Could you check a few things on this model? Use its own coordinates, in mm. A direction names the side the tool comes from. Give positions to 0.01 mm unless a question says otherwise; leave off trailing zeros. Loops run counter-clockwise (first coordinate to the right, second up) from the corner with the lowest first, then second, coordinate; pieces in that order, holes last. Notation, with made-up numbers: (84, 15) -> (96, 15) arc R5 ccw to (96, 21) -> close; hole circle Ø5 at (9.25, 14). An arc over 180 degrees is marked (long way). Write item = value, one per line. Start each with the question number.
1) I want a section at B-B (z = 0.5). List the corners of the cut face in (x, y) for me, and give its area (3 significant figures).
2) I want a section at A-A (y = 0). List the corners of the cut face in (x, z) for me.
3) I need wall thicknesses on probe 1 along Z at (x, y) = (6.5, 11); probe 2 along X at (y, z) = (-8.5, -0.7); probe 3 along X at (y, z) = (3, -1.5). Which ranges of each line are inside material? Lowest first, please. Write a range as from..to.
4) I'm going to push flat-ended pins straight in: pin 1 Ø1 at (x, z) = (1.5, -1) entering from +Y; pin 2 Ø0.6 at (x, z) = (-1, 1.5) entering from +Y. Where does each tip first touch, or does it pass through?
5) I want a section at C-C (x = -8). List the corners of the cut face in (y, z) for me, and give its area (3 significant figures).
6) On a 3-axis mill with a long thin cutter (end or side, diameter ignored), from which of +Z, -Z, +X, -X, +Y, -Y can I reach the whole of each face in a straight line? I mean faces 1 (the face through (3.09, 4.75, -0.94)), 2 (the face through (-11.811, -2.346, -0.937)), 3 (the face through (-5.88, 10.51, -0.94)), 4 (the face through (12.35, 0.37, -0.94)). Say none if no direction works.
7) I want a section at D-D (y = 8.5). List the corners of the cut face in (x, z) for me.
8) If we mould it in two halves opening along X, with no side actions, what happens to faces 5 (the face through (-4.518, 3.136, -0.937)), 6 (the face through (-9.774, -7.56, -0.937)), 7 (the face through (-7, 6, -1.9))? For each: +X half, -X half, draft (parallel to the pull), parting line (faces both ways), or undercut.
from build123d import *

# Parameters (mm, degrees)
SKETCH1_R           = 15.5
BOSS_EXTRUDE1_DEPTH = 2
BOSS_EXTRUDE2_DEPTH = 1.9
CIRPATTERN1_COUNT   = 5
CUT_EXTRUDE2_DEPTH  = 4.9


with BuildPart() as part:
    # Sketch1 → Boss-Extrude1 (new body)
    with BuildSketch(Plane.XY):
        Circle(SKETCH1_R)
    extrude(amount=BOSS_EXTRUDE1_DEPTH)

    # Sketch2 → Boss-Extrude2 (add)
    with BuildSketch(Plane(origin=(0, 0, 0), x_dir=(-1, 0, 0), z_dir=(0, 0, -1))):
        with BuildLine():
            Line((-7.817353518, 8.129035943), (-3.552701535, 4.927044661))
            ThreePointArc((-3.552701535, 4.927044661), (-3.081541521, 4.749426556), (-2.588715364, 4.852685109))
            ThreePointArc((-2.588715364, 4.852685109), (-1.571286021, 5.27077416), (-0.491007267, 5.478039053))
            ThreePointArc((-0.491007267, 5.478039053), (-0.022087339, 5.66148946), (0.274905404, 6.068103848))
            Line((0.274905404, 6.068103848), (2.090121325, 11.082582471))
            ThreePointArc((2.090121325, 11.082582471), (2.007658151, 11.864965509), (1.341576089, 12.283603874))
            ThreePointArc((1.341576089, 12.283603874), (-3.530150602, 11.841654752), (-7.848632729, 9.543883635))
            ThreePointArc((-7.848632729, 9.543883635), (-8.176755455, 8.82885995), (-7.817353518, 8.129035943))
        make_face()
    boss_extrude2 = extrude(amount=BOSS_EXTRUDE2_DEPTH)

    # CirPattern1: Boss-Extrude2 ×5 about axis
    cirpattern1_axis = Axis((0, 0, 0), (0, 0, 1))
    for i in range(1, CIRPATTERN1_COUNT):
        add(boss_extrude2.rotate(cirpattern1_axis, i * 360 / CIRPATTERN1_COUNT))

    # Sketch5 → Cut-Extrude2 (cut, through all)
    with BuildSketch(Plane.XY.offset(2)):
        with BuildLine():
            Line((-2.078460969, 1.95), (2.078460969, 1.95))
            ThreePointArc((2.078460969, 1.95), (2.85, 0), (2.078460969, -1.95))
            Line((2.078460969, -1.95), (-2.078460969, -1.95))
            ThreePointArc((-2.078460969, -1.95), (-2.85, 0), (-2.078460969, 1.95))
        make_face()
    extrude(amount=-CUT_EXTRUDE2_DEPTH, mode=Mode.SUBTRACT)


solid = part.part
Answer list:
q1.outline = circle Ø31 at (0, 0); hole (-2.08, -1.95) -> (2.08, -1.95) arc R2.85 ccw to (2.08, 1.95) -> (-2.08, 1.95) arc R2.85 ccw to start
q1.area = 734 mm^2
q2.outline = (-15.5, 0) -> (-2.85, 0) -> (-2.85, 2) -> (-15.5, 2) -> close; (2.85, 0) -> (5.5, 0) -> (5.5, -1.9) -> (12.36, -1.9) -> (12.36, 0) -> (15.5, 0) -> (15.5, 2) -> (2.85, 2) -> close
q3.probe_1 = 0..2
q3.probe_2 = -8.97..-4.33, -0.72..8.6
q3.probe_3 = -11.99..-4.61, 6.8..11.99
q4.pin_1 = 12.32
q4.pin_2 = 15.48
q5.outline = (-13.28, 0) -> (-9.42, 0) -> (-9.42, -1.9) -> (-1.93, -1.9) -> (-1.93, 0) -> (1.54, 0) -> (1.54, -1.9) -> (9.42, -1.9) -> (9.42, 0) -> (13.28, 0) -> (13.28, 2) -> (-13.28, 2) -> close
q5.area = 82.3 mm^2
q6.face_1 = -Z
q6.face_2 = -Z, -X
q6.face_3 = -Z, +Y
q6.face_4 = -Z, +X
q7.outline = (-12.96, 0) -> (-8.97, 0) -> (-8.97, -1.9) -> (-4.82, -1.9) -> (-4.82, 0) -> (-1.16, 0) -> (-1.16, -1.9) -> (8.11, -1.9) -> (8.11, 0) -> (12.96, 0) -> (12.96, 2) -> (-12.96, 2) -> close
q8.face_5 = undercut
q8.face_6 = -X half
q8.face_7 = draft
